Model file for the job. Use its own axes, mm. A direction names the side the tool comes from. Coordinates: 2 decimals unless noted, no trailing zeros. Order: outer loops, then holes, each group sorted by start corner. A loop starts at its lowest first (then second) coordinate and runs counter-clockwise, first axis right, second up. Notation, with made-up numbers: M 65.5,27.5 L 71.5,27.5 A28 cw 71.5,58.5 Z; hole C -20,35 d2. An arc over 180 degrees is marked long. Return JSON: item names as keys, results as strings.
Autodesk Fusion 360 part; units mm, degrees
sketch "Sketch2" plane through (0, 0, 0) normal (0, 0, 1) x (1, 0, 0)
  line L0 (0, 0) -> (100, 0)
  line L1 (100, 0) -> (100, 100)
  line L2 (100, 100) -> (0, 100)
  line L3 (0, 100) -> (0, 0)
extrude "Extrude3" add sketch "Sketch2" along normal blind 20
sketch "Sketch3" plane through (0, 0, 20) normal (0, 0, 1) x (-1, 0, 0)
  line L0 (0, -100) -> (0, 0)
  line L1 (0, 0) -> (-100, 0)
  line L2 (-100, 0) -> (-100, -100)
  line L3 (-100, -100) -> (0, -100)
  line L4 (-10, -10) -> (-90, -10)
  line L5 (-90, -10) -> (-90, -90)
  line L6 (-90, -90) -> (-10, -90)
  line L7 (-10, -90) -> (-10, -10)
extrude "Extrude4" cut sketch "Sketch3" against normal blind 10 contours L4 L5 L6 L7
sketch "Sketch4" plane through (0, 0, 10) normal (0, 0, 1) x (-1, 0, 0)
  line L0 (-10, -90) -> (-10, -10)
  line L1 (-10, -10) -> (-90, -10)
  line L2 (-90, -10) -> (-90, -90)
  line L3 (-90, -90) -> (-10, -90)
  spline S0 degree 3 poles (-75.4628, -68.295) (-73.8753, -68.1891) (-73.6636, -68.1362) (-73.5313, -67.6071) knots 0 0 0 0 1 1 1 1
  spline S1 degree 3 poles (-73.5313, -67.6071) (-72.473, -63.0562) (-68.3455, -46.4404) (-68.1338, -45.8583) knots 0 0 0 0 1 1 1 1
  spline S2 degree 3 poles (-68.1338, -45.8583) (-67.7369, -44.7471) (-64.7736, -31.8618) (-64.5355, -30.3008) knots 0 0 0 0 1 1 1 1
  spline S3 degree 3 poles (-64.5355, -30.3008) (-64.3503, -28.8456) (-64.0063, -28.8456) (-63.8211, -30.3273) knots 0 0 0 0 1 1 1 1
  spline S4 degree 3 poles (-63.8211, -30.3273) (-63.7417, -30.8829) (-62.4453, -34.6929) (-60.9371, -38.7939) knots 0 0 0 0 1 1 1 1
  line L4 (-60.9371, -38.7939) -> (-58.1855, -46.2552)
  line L5 (-58.1855, -46.2552) -> (-55.4073, -46.2552)
  line L6 (-55.4073, -46.2552) -> (-52.6028, -46.2552)
  line L7 (-52.6028, -46.2552) -> (-50.0363, -38.4764)
  spline S5 degree 3 poles (-50.0363, -38.4764) (-48.634, -34.2166) (-47.4698, -30.4596) (-47.4698, -30.1421) knots 0 0 0 0 1 1 1 1
  spline S6 degree 3 poles (-47.4698, -30.1421) (-47.4698, -29.0308) (-46.9936, -29.6129) (-46.8348, -30.9887) knots 0 0 0 0 1 1 1 1
  spline S7 degree 3 poles (-46.8348, -30.9887) (-46.729, -31.7296) (-45.9882, -35.275) (-45.1944, -38.8204) knots 0 0 0 0 1 1 1 1
  line L8 (-45.1944, -38.8204) -> (-43.7657, -45.2762)
  line L9 (-43.7657, -45.2762) -> (-44.824, -46.1758)
  spline S8 degree 3 poles (-44.824, -46.1758) (-46.3057, -47.4723) (-47.1523, -49.0333) (-47.6021, -51.4146) knots 0 0 0 0 1 1 1 1
  spline S9 degree 3 poles (-47.6021, -51.4146) (-48.0784, -53.7958) (-48.1048, -55.8066) (-47.708, -58.1614) knots 0 0 0 0 1 1 1 1
  spline S10 degree 3 poles (-47.708, -58.1614) (-47.1788, -61.5216) (-45.7765, -63.6648) (-43.263, -65.0141) knots 0 0 0 0 1 1 1 1
  spline S11 degree 3 poles (-43.263, -65.0141) (-40.8288, -66.3106) (-38.5269, -66.6281) (-31.833, -66.6281) knots 0 0 0 0 1 1 1 1
  line L10 (-31.833, -66.6281) -> (-26.0386, -66.6281)
  line L11 (-26.0386, -66.6281) -> (-26.0386, -44.8)
  line L12 (-26.0386, -44.8) -> (-26.0386, -22.9718)
  line L13 (-26.0386, -22.9718) -> (-29.2136, -22.9718)
  line L14 (-29.2136, -22.9718) -> (-32.3886, -22.9718)
  line L15 (-32.3886, -22.9718) -> (-32.3886, -33.2377)
  line L16 (-32.3886, -33.2377) -> (-32.3886, -43.4771)
  line L17 (-32.3886, -43.4771) -> (-34.6905, -43.4241)
  line L18 (-34.6905, -43.4241) -> (-36.9659, -43.3712)
  line L19 (-36.9659, -43.3712) -> (-39.7969, -33.2377)
  line L20 (-39.7969, -33.2377) -> (-42.6015, -23.1041)
  line L21 (-42.6015, -23.1041) -> (-45.803, -23.0248)
  line L22 (-45.803, -23.0248) -> (-48.978, -22.9454)
  line L23 (-48.978, -22.9454) -> (-51.6503, -30.83)
  spline S12 degree 3 poles (-51.6503, -30.83) (-53.1319, -35.1691) (-54.4019, -39.085) (-54.5078, -39.5083) knots 0 0 0 0 1 1 1 1
  spline S13 degree 3 poles (-54.5078, -39.5083) (-54.8517, -41.1752) (-54.9311, -41.3339) (-55.1692, -40.9371) knots 0 0 0 0 1 1 1 1
  spline S14 degree 3 poles (-55.1692, -40.9371) (-55.3015, -40.7254) (-55.4073, -40.355) (-55.4073, -40.0904) knots 0 0 0 0 1 1 1 1
  spline S15 degree 3 poles (-55.4073, -40.0904) (-55.4073, -39.8258) (-56.8096, -35.8835) (-58.503, -31.3062) knots 0 0 0 0 1 1 1 1
  line L24 (-58.503, -31.3062) -> (-61.5986, -22.9983)
  line L25 (-61.5986, -22.9983) -> (-65.144, -22.9189)
  spline S16 degree 3 poles (-65.144, -22.9189) (-67.1019, -22.866) (-68.7159, -22.8925) (-68.7688, -22.9718) knots 0 0 0 0 1 1 1 1
  spline S17 degree 3 poles (-68.7688, -22.9718) (-68.8482, -23.1306) (-79.749, -68.1098) (-79.749, -68.3214) knots 0 0 0 0 1 1 1 1
  spline S18 degree 3 poles (-79.749, -68.3214) (-79.749, -68.4802) (-79.0346, -68.4802) (-75.4628, -68.295) knots 0 0 0 0 1 1 1 1
  spline S19 degree 3 poles (-78.1615, -66.6546) (-78.1615, -66.0989) (-68.1603, -24.6123) (-67.9486, -24.2683) knots 0 0 0 0 1 1 1 1
  spline S20 degree 3 poles (-67.9486, -24.2683) (-67.7105, -23.8714) (-62.6569, -23.9773) (-62.3394, -24.3741) knots 0 0 0 0 1 1 1 1
  spline S21 degree 3 poles (-62.3394, -24.3741) (-62.1807, -24.5329) (-60.8048, -28.1577) (-59.2438, -32.3646) knots 0 0 0 0 1 1 1 1
  spline S22 degree 3 poles (-59.2438, -32.3646) (-56.1217, -40.8841) (-55.9894, -41.1752) (-55.3544, -41.5985) knots 0 0 0 0 1 1 1 1
  spline S23 degree 3 poles (-55.3544, -41.5985) (-54.4548, -42.1541) (-53.8992, -40.9635) (-51.3063, -33.026) knots 0 0 0 0 1 1 1 1
  spline S24 degree 3 poles (-51.3063, -33.026) (-49.904, -28.7398) (-48.5811, -24.9562) (-48.3694, -24.6123) knots 0 0 0 0 1 1 1 1
  spline S25 degree 3 poles (-48.3694, -24.6123) (-48.0255, -24.0831) (-47.7873, -24.0302) (-45.7765, -24.0302) knots 0 0 0 0 1 1 1 1
  spline S26 degree 3 poles (-45.7765, -24.0302) (-43.6069, -24.0302) (-43.554, -24.0566) (-43.2894, -24.7446) knots 0 0 0 0 1 1 1 1
  spline S27 degree 3 poles (-43.2894, -24.7446) (-43.1307, -25.1679) (-41.8871, -29.4541) (-40.5642, -34.3225) knots 0 0 0 0 1 1 1 1
  spline S28 degree 3 poles (-40.5642, -34.3225) (-39.1884, -39.2702) (-37.8919, -43.4241) (-37.6009, -43.7681) knots 0 0 0 0 1 1 1 1
  spline S29 degree 3 poles (-37.6009, -43.7681) (-37.1511, -44.3502) (-36.913, -44.4031) (-34.7963, -44.4031) knots 0 0 0 0 1 1 1 1
  spline S30 degree 3 poles (-34.7963, -44.4031) (-31.2244, -44.4031) (-31.489, -45.1968) (-31.3303, -33.7139) knots 0 0 0 0 1 1 1 1
  line L26 (-31.3303, -33.7139) -> (-31.198, -24.1625)
  line L27 (-31.198, -24.1625) -> (-29.3723, -24.0831)
  spline S31 degree 3 poles (-29.3723, -24.0831) (-28.0759, -24.0302) (-27.4673, -24.1096) (-27.3351, -24.3477) knots 0 0 0 0 1 1 1 1
  spline S32 degree 3 poles (-27.3351, -24.3477) (-27.0705, -24.7446) (-27.0176, -64.5114) (-27.2557, -65.1464) knots 0 0 0 0 1 1 1 1
  spline S33 degree 3 poles (-27.2557, -65.1464) (-27.4938, -65.755) (-36.5426, -65.755) (-39.4794, -65.1464) knots 0 0 0 0 1 1 1 1
  spline S34 degree 3 poles (-39.4794, -65.1464) (-44.7976, -64.0616) (-46.8084, -61.2835) (-46.8084, -54.9864) knots 0 0 0 0 1 1 1 1
  spline S35 degree 3 poles (-46.8084, -54.9864) (-46.7819, -50.7531) (-46.2263, -49.1391) (-43.9244, -46.705) knots 0 0 0 0 1 1 1 1
  spline S36 degree 3 poles (-43.9244, -46.705) (-43.2365, -45.9641) (-42.9719, -45.4614) (-42.9719, -44.8529) knots 0 0 0 0 1 1 1 1
  spline S37 degree 3 poles (-42.9719, -44.8529) (-42.9719, -44.3766) (-43.6598, -40.8841) (-44.533, -37.0477) knots 0 0 0 0 1 1 1 1
  spline S38 degree 3 poles (-44.533, -37.0477) (-45.7236, -31.6502) (-46.1998, -29.9568) (-46.6232, -29.5071) knots 0 0 0 0 1 1 1 1
  spline S39 degree 3 poles (-46.6232, -29.5071) (-47.1788, -28.9779) (-47.2053, -28.9779) (-47.708, -29.4277) knots 0 0 0 0 1 1 1 1
  spline S40 degree 3 poles (-47.708, -29.4277) (-48.0519, -29.7187) (-49.0573, -32.391) (-50.4067, -36.4391) knots 0 0 0 0 1 1 1 1
  spline S41 degree 3 poles (-50.4067, -36.4391) (-51.5973, -40.011) (-52.788, -43.4506) (-53.0526, -44.0856) knots 0 0 0 0 1 1 1 1
  line L28 (-53.0526, -44.0856) -> (-53.5553, -45.2233)
  line L29 (-53.5553, -45.2233) -> (-55.4603, -45.1439)
  line L30 (-55.4603, -45.1439) -> (-57.3917, -45.0646)
  line L31 (-57.3917, -45.0646) -> (-58.0267, -43.4771)
  spline S42 degree 3 poles (-58.0267, -43.4771) (-58.3707, -42.6039) (-59.6936, -39.0321) (-60.9901, -35.5396) knots 0 0 0 0 1 1 1 1
  spline S43 degree 3 poles (-60.9901, -35.5396) (-62.2865, -32.0471) (-63.5301, -29.0308) (-63.7946, -28.8721) knots 0 0 0 0 1 1 1 1
  spline S44 degree 3 poles (-63.7946, -28.8721) (-64.1386, -28.581) (-64.3238, -28.6075) (-64.7207, -28.9779) knots 0 0 0 0 1 1 1 1
  spline S45 degree 3 poles (-64.7207, -28.9779) (-65.2763, -29.4806) (-65.3821, -29.851) (-66.6521, -35.275) knots 0 0 0 0 1 1 1 1
  spline S46 degree 3 poles (-66.6521, -35.275) (-67.6311, -39.5348) (-68.6894, -43.7946) (-69.9594, -48.6364) knots 0 0 0 0 1 1 1 1
  spline S47 degree 3 poles (-69.9594, -48.6364) (-70.3828, -50.3033) (-71.5205, -54.96) (-72.4994, -58.9552) knots 0 0 0 0 1 1 1 1
  spline S48 degree 3 poles (-72.4994, -58.9552) (-73.4519, -62.9504) (-74.3515, -66.4429) (-74.4838, -66.7075) knots 0 0 0 0 1 1 1 1
  spline S49 degree 3 poles (-74.4838, -66.7075) (-74.6955, -67.0514) (-75.0923, -67.1573) (-76.4417, -67.1573) knots 0 0 0 0 1 1 1 1
  spline S50 degree 3 poles (-76.4417, -67.1573) (-77.9498, -67.1573) (-78.1615, -67.1043) (-78.1615, -66.6546) knots 0 0 0 0 1 1 1 1
  spline S51 degree 3 poles (-32.759, -63.215) (-31.4096, -62.6329) (-31.3303, -62.236) (-31.3303, -55.1981) knots 0 0 0 0 1 1 1 1
  spline S52 degree 3 poles (-31.3303, -55.1981) (-31.3303, -50.9648) (-31.4361, -48.4248) (-31.6213, -48.0279) knots 0 0 0 0 1 1 1 1
  spline S53 degree 3 poles (-31.6213, -48.0279) (-32.124, -46.9431) (-32.9178, -46.705) (-35.4842, -46.8373) knots 0 0 0 0 1 1 1 1
  spline S54 degree 3 poles (-35.4842, -46.8373) (-40.0615, -47.1018) (-42.0194, -48.7952) (-42.7338, -53.0814) knots 0 0 0 0 1 1 1 1
  spline S55 degree 3 poles (-42.7338, -53.0814) (-43.1042, -55.3039) (-42.7338, -58.3996) (-41.9401, -59.9871) knots 0 0 0 0 1 1 1 1
  spline S56 degree 3 poles (-41.9401, -59.9871) (-41.2521, -61.31) (-39.7969, -62.5535) (-38.5534, -62.8975) knots 0 0 0 0 1 1 1 1
  spline S57 degree 3 poles (-38.5534, -62.8975) (-37.1246, -63.3208) (-33.4205, -63.506) (-32.759, -63.215) knots 0 0 0 0 1 1 1 1
  spline S58 degree 3 poles (-38.2359, -61.8656) (-39.6911, -61.4687) (-40.9876, -60.1723) (-41.4109, -58.6641) knots 0 0 0 0 1 1 1 1
  spline S59 degree 3 poles (-41.4109, -58.6641) (-41.5961, -58.0291) (-41.7548, -56.3093) (-41.7548, -54.8277) knots 0 0 0 0 1 1 1 1
  spline S60 degree 3 poles (-41.7548, -54.8277) (-41.7548, -52.5523) (-41.649, -51.9966) (-41.0934, -50.8589) knots 0 0 0 0 1 1 1 1
  spline S61 degree 3 poles (-41.0934, -50.8589) (-40.0351, -48.7158) (-38.0771, -47.8427) (-34.2407, -47.8427) knots 0 0 0 0 1 1 1 1
  line L32 (-34.2407, -47.8427) -> (-32.3886, -47.8427)
  line L33 (-32.3886, -47.8427) -> (-32.3886, -55.0923)
  line L34 (-32.3886, -55.0923) -> (-32.3886, -62.3418)
  line L35 (-32.3886, -62.3418) -> (-34.7434, -62.2625)
  spline S62 degree 3 poles (-34.7434, -62.2625) (-36.0398, -62.2096) (-37.6009, -62.0243) (-38.2359, -61.8656) knots 0 0 0 0 1 1 1 1
extrude "Extrude5" add sketch "Sketch4" along normal blind 5 contours S19 S20 S21 S22 S23 S24 S25 S26 S27 S28 S29 S30 L26 L27 S31 S32 S33 S34 S35 S36 S37 S38 S39 S40 S41 L28 L29 L30 L31 S42 S43 S44 S45 S46 S47 S48 S49 S50
Item 1: Saw through at B-B (y = 17.5). Write the cut outline in (x, z), and give its area (3 significant figures).
Check result:
{"outline": "M 0,0 L 100,0 L 100,20 L 90,20 L 90,10 L 10,10 L 10,20 L 0,20 Z", "area": "1,200 mm2"}
Item 2: 3-axis set-ups, long thin cutter, end or side, ignore diameter. For faces 4 (the flat face through (90, 49, 15)), 5 (the flat face through (100, 49, 10)): which of +Z, -Z, +X, -X, +Y, -Y reach the whole face in a straight line?
Check result:
{"face 4": "+Z", "face 5": "+Z, -Z, +X, +Y, -Y"}
Item 3: Saw through at A-A (z = 16.75). Write the cut outline in (x, y), and give its area (3 significant figures).
Check result:
{"outline": "M 0,0 L 100,0 L 100,100 L 0,100 Z; hole M 10,10 L 90,10 L 90,90 L 10,90 Z", "area": "3,600 mm2"}
Item 4: Pull direction Y, two halves, no side cores. Call faces 1 (the flat face through (0, 51, 10)), 2 (the flat face through (49, 0, 10)), 3 (the flat face through (10, 51, 15)): +Y half, -Y half, draft (parallel to the pull), parting line (faces both ways), or undercut.
Check result:
{"face 1": "draft", "face 2": "-Y half", "face 3": "undercut"}
Item 5: Drop flat-ended pins along their axis: pin 1 Ø13 at (x, y) = (40.5, 48) entering from +Z; pin 2 Ø4 at (x, y) = (12.5, 68.5) entering from +Z. Give the stop position or say it passes through.
Check result:
{"pin 1": "stops at z = 15", "pin 2": "stops at z = 10"}
Item 6: Wall check: line 1 (X direction, y = 47, z = 19); line 2 (Z direction, x = 50, y = 40). Give the ranges that are in metal, low to high.
Check result:
{"line 1": "x = 0 to 10, 90 to 100", "line 2": "z = 0 to 10"}
